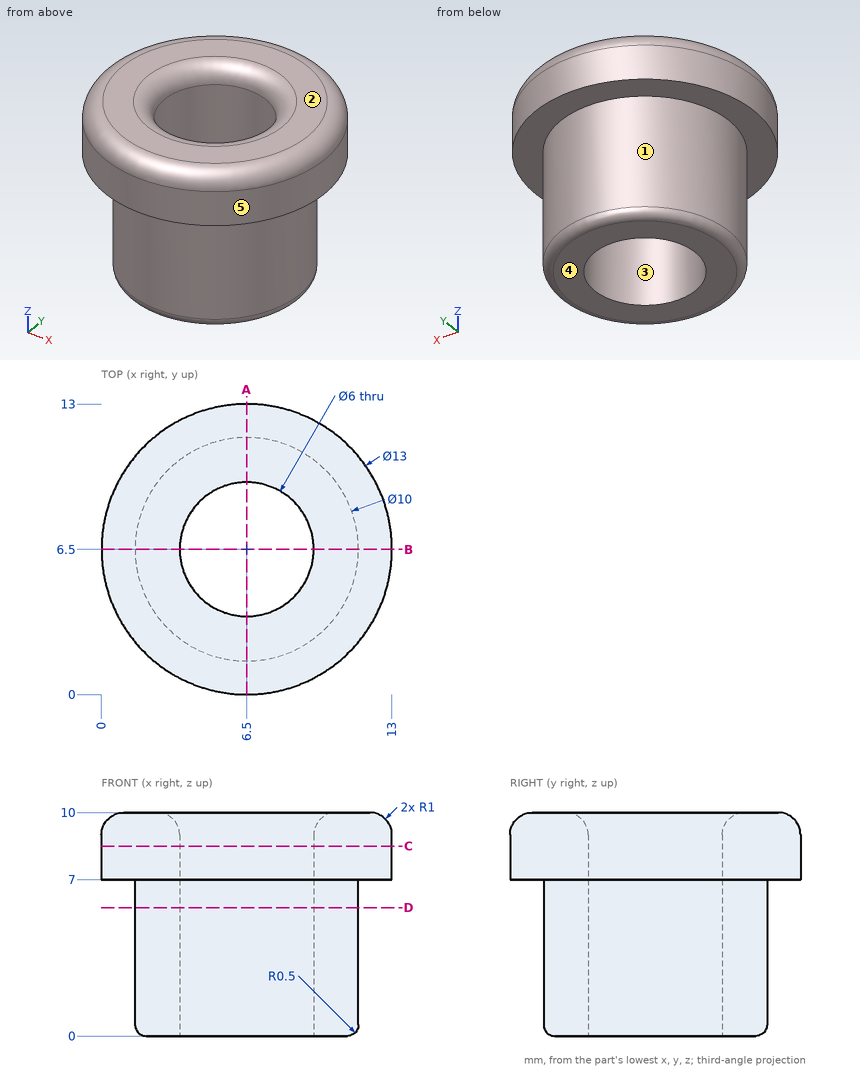
Print and shaded views of the part. All mm, measured from the part's lowest x, y and z. A direction names the side the tool comes from. Coordinates: 2 decimals unless noted, no trailing zeros. Write each loop counter-clockwise with the first axis right and the second up, starting at its lowest first coordinate (ties: lowest second). Pieces come first, ordered by that corner, then holes.
(1) Cut at D-D, the plane z = 5.75. List the corners of the cut face in (x, y).
(2) 3-axis set-ups, long thin cutter, end or side, ignore diameter. For the marked faces 1 and 2: which of +Z, -Z, +X, -X, +Y, -Y reach the whole face in a straight line?
(3) Two-plate mould, pull along Y, no slides. Class the marked faces 3, 4 and 5: +Y half, -Y half, draft (parallel to the pull), parting line (faces both ways), or undercut.
(4) Cut at A-A, the plane x = 6.5. List the corners of the cut face in (y, z), and give its area (3 significant figures).
(5) Cut at C-C, the plane z = 8.5. List the corners of the cut face in (x, y).
(6) Flat gauge pins, fed straight in: pin 1 (5 mm diameter, centred on x = 6.5, y = 6.5, fed in from +Z); pin 2 (2 mm diameter, centred on x = 8, z = 1.5, fed in from -Y); pin 3 (4 mm diameter, centred on y = 1.5, z = 3, fed in from +X); pin 4 (2 mm diameter, centred on x = 1.5, z = 1.5, fed in from -Y). Where does each tip first touch, or does it go through?
(7) Drill centre lines: probe 1 along Y at (x, z) = (6.5, 3.75); probe 2 along Y at (x, z) = (6.5, 7.25); probe 3 along Z at (x, y) = (11.5, 9). Where is each one in solid material? Low to high.
Geometry says:
1. outline: circle Ø10 at (6.5, 6.5); hole circle Ø6 at (6.5, 6.5)
2. face 1: -Z
2. face 2: +Z, +X, -X, +Y, -Y
3. face 3: undercut
3. face 4: draft
3. face 5: parting line
4. outline: (0, 7) - (1.5, 7) - (1.5, 0.5) arc R0.5 ccw to (2, 0) - (3.5, 0) - (3.5, 9) arc R1 ccw to (2.5, 10) - (1, 10) arc R1 ccw to (0, 9) - close; (9.5, 0) - (11, 0) arc R0.5 ccw to (11.5, 0.5) - (11.5, 7) - (13, 7) - (13, 9) arc R1 ccw to (12, 10) - (10.5, 10) arc R1 ccw to (9.5, 9) - close
4. area: 48.0 mm2
5. outline: circle Ø13 at (6.5, 6.5); hole circle Ø6 at (6.5, 6.5)
6. pin 1: passes through
6. pin 2: stops at y = 1.53
6. pin 3: stops at x = 10.5
6. pin 4: stops at y = 3.5
7. probe 1: y = 1.5 to 3.5, 9.5 to 11.5
7. probe 2: y = 0 to 3.5, 9.5 to 13
7. probe 3: z = 7 to 10
